```python
from build123d import *

# Parameters (mm, degrees)
BOSS_EXTRUDE1_DEPTH = 20
SKETCH2_R           = 10
CUT_EXTRUDE1_DEPTH  = 77.47875522
SKETCH6_R           = 2.75
CUT_EXTRUDE2_DEPTH  = 10


with BuildPart() as part:
    # Sketch1 → Boss-Extrude1 (new body)
    with BuildSketch(Plane(origin=(0, 0, 0), x_dir=(1, 0, 0), z_dir=(0, 1, 0))):
        Polygon((0, 32.5), (0, 0), (60, 0), (60, 32.5), (43.75, 32.5), (43.75, 43), (16.25, 43), (16.25, 32.5), align=None)
    extrude(amount=BOSS_EXTRUDE1_DEPTH)

    # Sketch2 → Cut-Extrude1 (cut, through all)
    with BuildSketch(Plane(origin=(0, 20, 0), x_dir=(1, 0, 0), z_dir=(0, 1, 0))):
        with Locations(Location((30, 25, 0), (0, 0, 270))):
            Circle(SKETCH2_R)
    extrude(amount=-CUT_EXTRUDE1_DEPTH, mode=Mode.SUBTRACT)

    # Sketch6 → Cut-Extrude2 (cut)
    with BuildSketch(Plane.XY):
        with Locations((7, 10)):
            Circle(SKETCH6_R)
        with Locations((53, 10)):
            Circle(SKETCH6_R)
    extrude(amount=-CUT_EXTRUDE2_DEPTH, mode=Mode.SUBTRACT)


solid = part.part
```
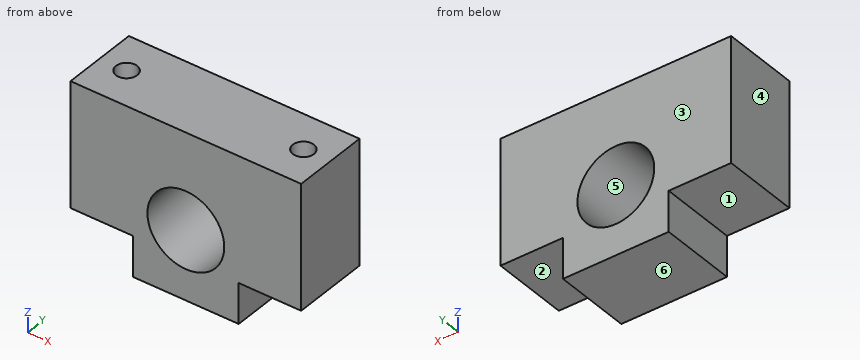
Verification items for the finished model (mm, model axes). Face numbers are marked on the shaded views. A direction names the side the tool comes from. Give positions to 0.01 mm unless a question says otherwise; leave off trailing zeros. Order: outer loops, then holes, each group sorted by start corner. A loop starts at its lowest first (then second) coordinate and runs counter-clockwise, first axis right, second up. Notation, with made-up numbers: M 43,43.25 L 69,43.25 A15 cw 69,57.25 Z; hole C 23,50 d3. An arc over 180 degrees is marked long. Answer in a Markdown table with one row per item. Add a question column.
Item 1: Section check B-B, the plane y = 10. Enter the section's corners in (x, z), and give its area (3 significant figures).
Item 2: Section check D-D, the plane y = 18.5. Enter the section's corners in (x, z), and give its area (3 significant figures).
Item 3: Section check A-A, the plane z = -25. Enter the section's corners in (x, y).
Item 4: Mould release check, pull along X, two halves, no side actions. Record for the marked faces 4, 5 and 6: released by +X, released by -X, zero draft, split by the parting line, or undercut.
Item 5: Gauge pin test, flat ends, axial feed: pin 1 (5 mm diameter, centred on y = 11, z = -40.5, fed in from -X); pin 2 (5 mm diameter, centred on y = 9, z = -35.5, fed in from +X); pin 3 (3.5 mm diameter, centred on x = 7, y = 10, fed in from +Z). Record the tip position at first contact, or that the pin passes through.
Item 6: Tool access check on the marked faces 1, 2 and 3. Record the directions out of +Z, -Z, +X, -X, +Y, -Y that give a thin tool (end or side, any length) a straight path to the whole face; none if there is none.
Item 7: Section check C-C, the plane x = 30. Enter the section's corners in (y, z), and give its area (3 significant figures).
Item 8: Scan lines: probe 1 along X at (y, z) = (14.5, -25); probe 2 along Y at (x, z) = (53, -5); probe 3 along X at (y, z) = (10.5, -9.5). Record each from-to range of solid material in increasing order. Write a range as from..to.
Filled sheet:
| question | item | result |
|---|---|---|
| 1 | outline | M 0,-32.5 L 16.25,-32.5 L 16.25,-43 L 43.75,-43 L 43.75,-32.5 L 60,-32.5 L 60,0 L 55.75,0 L 55.75,-10 L 50.25,-10 L 50.25,0 L 9.75,0 L 9.75,-10 L 4.25,-10 L 4.25,0 L 0,0 Z; hole C 30,-25 d20 |
| 1 | area | 1,810 mm^2 |
| 2 | outline | M 0,-32.5 L 16.25,-32.5 L 16.25,-43 L 43.75,-43 L 43.75,-32.5 L 60,-32.5 L 60,0 L 0,0 Z; hole C 30,-25 d20 |
| 2 | area | 1,920 mm^2 |
| 3 | outline | M 0,0 L 20,0 L 20,20 L 0,20 Z; M 40,0 L 60,0 L 60,20 L 40,20 Z |
| 4 | face 4 | released by -X |
| 4 | face 5 | undercut |
| 4 | face 6 | zero draft |
| 5 | pin 1 | stops at x = 16.25 |
| 5 | pin 2 | stops at x = 43.75 |
| 5 | pin 3 | stops at z = -10 |
| 6 | face 1 | -Z, -X, +Y, -Y |
| 6 | face 2 | -Z, +X, +Y, -Y |
| 6 | face 3 | +Z, -Z, +X, -X, +Y |
| 7 | outline | M 0,-43 L 20,-43 L 20,-35 L 0,-35 Z; M 0,-15 L 20,-15 L 20,0 L 0,0 Z |
| 7 | area | 460 mm^2 |
| 8 | probe 1 | x = 0..20, 40..60 |
| 8 | probe 2 | y = 0..7.25, 12.75..20 |
| 8 | probe 3 | x = 0..4.3, 9.7..50.3, 55.7..60 |
